Could you check a few things on this model? Use its own coordinates, in mm. Round coordinates to 2 decimals unless told otherwise and drop trailing zeros. Write each loop counter-clockwise with the first axis right and the second up, starting at its lowest first coordinate (ties: lowest second). Pieces come first, ordered by that corner, then holes.
```python
from build123d import *

# Parameters (mm, degrees)
F0_W     = 120
F0_H     = 90
F0_R     = 1
F0_R_2   = 5
F1_DEPTH = 3
F2_R     = 5
F2_R_2   = 1
F3_DEPTH = 3.001


with BuildPart() as f1:
    # F0 (on Top) → F1 (new body)
    with BuildSketch(Plane.XY):
        Rectangle(F0_W, F0_H)
        with Locations((-5.085, -18.47)):
            Circle(F0_R, mode=Mode.SUBTRACT)
        with Locations((5.09234, -18.47)):
            Circle(F0_R, mode=Mode.SUBTRACT)
        with Locations((0, -5)):
            Circle(F0_R_2, mode=Mode.SUBTRACT)
        with Locations((-5.085, 28.79)):
            Circle(F0_R, mode=Mode.SUBTRACT)
        with Locations((5.09234, 28.79)):
            Circle(F0_R, mode=Mode.SUBTRACT)
        with Locations((0, -5)):
            Circle(F0_R_2)
        with Locations((5.09234, 28.79)):
            Circle(F0_R)
        with Locations((-5.085, 28.79)):
            Circle(F0_R)
        with Locations((-5.085, -18.47)):
            Circle(F0_R)
        with Locations((5.09234, -18.47)):
            Circle(F0_R)
    extrude(amount=F1_DEPTH)

    # F2 (on face) → F3 (cut, through all)
    with BuildSketch(Plane.XY.offset(3)):
        with Locations((0, 5)):
            Circle(F2_R)
        with Locations((5.085, -28.79)):
            Circle(F2_R_2)
        with Locations((-5.085, -28.79)):
            Circle(F2_R_2)
        with Locations((5.085, 18.47)):
            Circle(F2_R_2)
        with Locations((-5.085, 18.47)):
            Circle(F2_R_2)
    extrude(amount=-F3_DEPTH, mode=Mode.SUBTRACT)


solid = f1.part
```
Q1. We'd pull the mould along X, two halves only. Please class faces 1 (the cylindrical face through (-1.08, 0.12, 1.52)), 2 (the flat face through (60, -1, 1)), 3 (the flat face through (-60, -1, 1)): pulls with the +X half, pulls with the -X half, needs draft (parallel to the pull), parting line crosses it, or undercut.
Q2. Imagine slicing it at A-A, the plane y = 5. Write out the boundary of the cut face in (x, z).
Q3. Imagine slicing it at B-B, the plane x = 0. Write out the boundary of the cut face in (y, z), then the cut area to 3 significant figures.
Q4. I'm going to push a flat-ended pin straight in: pin 1 Ø13 at (x, y) = (0, 5) entering from -Z. Where does the tip first touch, or does it pass through?
Q5. If I drill on L1, parallel to Y at x = 0, z = 2; L2, parallel to X at y = 6, z = 1.05; L3, parallel to Y at x = -4.5, z = 2.15, over which ranges is the centre line in solid material (lowest first)?
Results found:
1. face 1: undercut
1. face 2: pulls with the +X half
1. face 3: pulls with the -X half
2. outline: (-60, 0) - (-5, 0) - (-5, 3) - (-60, 3) - close; (5, 0) - (60, 0) - (60, 3) - (5, 3) - close
3. outline: (-45, 0) - (0, 0) - (0, 3) - (-45, 3) - close; (10, 0) - (45, 0) - (45, 3) - (10, 3) - close
3. area: 240 mm2
4. pin 1: stops at z = 0
5. L1: y = -45 to 0, 10 to 45
5. L2: x = -60 to -4.9, 4.9 to 60
5. L3: y = -45 to -29.6, -27.98 to 2.82, 7.18 to 17.66, 19.28 to 45
